Read the model definition and answer for the solid it produces. Units are mm, in the model's axes. Round coordinates to 2 decimals unless told otherwise and drop trailing zeros. Order: outer loops, then holes, each group sorted by start corner. A loop starts at its lowest first (then second) coordinate and runs counter-clockwise, first axis right, second up. Notation, with made-up numbers: (86.25, 69) -> (96.25, 69) arc R14 ccw to (96.25, 75) -> close; hole circle Ø10 at (50.25, -34). An arc over 180 degrees is marked (long way). One line per item, written item: value. Start each with the question number.
1. A flat-ended cylindrical pin translates along its axis: pin 1 Ø4 at (x, z) = (6.5, 7) entering from -Y. Find the tip coordinate at first contact, or state that the pin passes through.
2. Consider line 1 (Y direction, x = 18.75, z = 2.5); line 2 (Y direction, x = 5.75, z = 14); line 3 (X direction, y = 6.5, z = 2.5). Determine where each line is inside the solid, lowest interval first.
3. Section B-B (x = 16.5) is taken. Give the vertices of the cut face in (y, z).
4. Section C-C (x = 4.25) is taken. Give the vertices of the cut face in (y, z), then the cut area to 3 significant figures.
from build123d import *

# Parameters (mm, degrees)
ESQUISSE1_W        = 20
ESQUISSE1_H        = 110
BOSS_EXTRU_1_DEPTH = 20
CONG_3_R           = 10


with BuildPart() as part:
    # Esquisse1 → Boss.-Extru.1 (new body)
    with BuildSketch(Plane.XY):
        with Locations((10, 55)):
            Rectangle(ESQUISSE1_W, ESQUISSE1_H)
    extrude(amount=BOSS_EXTRU_1_DEPTH)

    # Congé3
    cong_3_edges = [part.edges().sort_by_distance(p)[0] for p in [
        (0, 0, 10),
        (20, 0, 10),
    ]]
    fillet(cong_3_edges, radius=CONG_3_R - 0.0001)  # a hair under: the kernel refuses the full size


solid = part.part
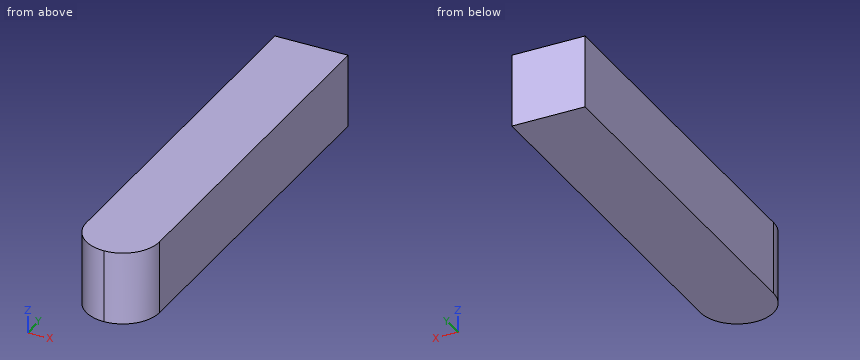
Answer:
1. pin 1: y = 0.11
2. line 1: 5.16 to 110
2. line 2: 0.95 to 110
2. line 3: 0.63 to 19.37
3. outline: (2.4, 0) -> (110, 0) -> (110, 20) -> (2.4, 20) -> close
4. outline: (1.82, 0) -> (110, 0) -> (110, 20) -> (1.82, 20) -> close
4. area: 2,160 mm^2
